Check sheet for the modelled part. Datum: model origin and axes. Units: mm. Face numbers are marked on the shaded views. A direction names the side the tool comes from. Give positions to 0.01 mm unless a question says otherwise; leave off trailing zeros. Order: outer loops, then holes, each group sorted by start corner. A loop starts at its lowest first (then second) coordinate and runs counter-clockwise, first axis right, second up. Notation, with made-up numbers: (-33, 85.5) - (-14, 85.5) arc R18 ccw to (-14, 116.5) - close; hole circle Ø11 at (-33.75, 56.5). An arc over 180 degrees is marked (long way). Answer in a Markdown table with one row per item.
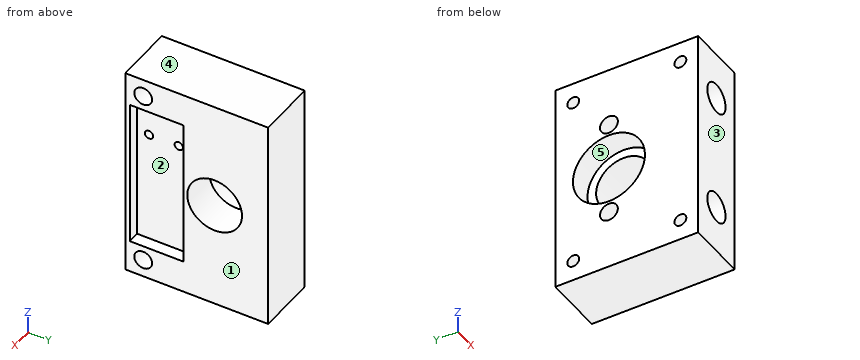
from build123d import *

# Parameters (mm, degrees)
SKETCH_1_W           = 36
SKETCH_1_H           = 24
EXTRUDE_1_DEPTH      = 10
SKETCH_2_R           = 6.05
CUT_EXTRUDE_1_DEPTH  = 4
SKETCH_3_R           = 4.6
CUT_EXTRUDE_2_DEPTH  = 7
SKETCH_5_R           = 2.5
CUT_EXTRUDE_4_DEPTH  = 8
SKETCH_7_W           = 25
SKETCH_7_H           = 9
CUT_EXTRUDE_5_DEPTH  = 2
SKETCH_8_R           = 1.5
CUT_EXTRUDE_6_DEPTH  = 5
SKETCH_9_R           = 1.5
CUT_EXTRUDE_7_DEPTH  = 5
SKETCH_11_R          = 1
CUT_EXTRUDE_9_DEPTH  = 3
SKETCH_13_R          = 0.7
CUT_EXTRUDE_10_DEPTH = 5


with BuildPart() as part:
    # 草图1 → 凸台-拉伸1 (new body)
    with BuildSketch(Plane(origin=(0, 0, 0), x_dir=(0, 0, -1), z_dir=(1, 0, 0))):
        with Locations((18, -12)):
            Rectangle(SKETCH_1_W, SKETCH_1_H)
    extrude(amount=EXTRUDE_1_DEPTH)

    # 草图2 → 切除-拉伸1 (cut)
    with BuildSketch(Plane.ZY):
        with Locations((-18, -9)):
            Circle(SKETCH_2_R)
    extrude(amount=-CUT_EXTRUDE_1_DEPTH, mode=Mode.SUBTRACT)

    # 草图3 → 切除-拉伸2 (cut, through all)
    with BuildSketch(Plane.ZY.offset(-4)):
        with Locations((-18, -9)):
            Circle(SKETCH_3_R)
    extrude(amount=-CUT_EXTRUDE_2_DEPTH, mode=Mode.SUBTRACT)

    # 草图5 → 切除-拉伸4 (cut)
    with BuildSketch(Plane(origin=(0, -24, 0), x_dir=(-1, 0, 0), z_dir=(0, -1, 0))):
        with Locations((-5, 28)):
            Circle(SKETCH_5_R)
        with Locations((-5, 8)):
            Circle(SKETCH_5_R)
    extrude(amount=-CUT_EXTRUDE_4_DEPTH, mode=Mode.SUBTRACT)

    # 草图7 → 切除-拉伸5 (cut)
    with BuildSketch(Plane(origin=(10, 0, 0), x_dir=(0, 0, -1), z_dir=(1, 0, 0))):
        with Locations((18, -18.75)):
            Rectangle(SKETCH_7_W, SKETCH_7_H)
    extrude(amount=-CUT_EXTRUDE_5_DEPTH, mode=Mode.SUBTRACT)

    # 草图8 → 切除-拉伸6 (cut)
    with BuildSketch(Plane.ZY):
        with Locations((-10, -9)):
            Circle(SKETCH_8_R)
        with Locations((-26, -9)):
            Circle(SKETCH_8_R)
    extrude(amount=-CUT_EXTRUDE_6_DEPTH, mode=Mode.SUBTRACT)

    # 草图9 → 切除-拉伸7 (cut)
    with BuildSketch(Plane(origin=(10, 0, 0), x_dir=(0, 0, -1), z_dir=(1, 0, 0))):
        with Locations((3, -21)):
            Circle(SKETCH_9_R)
        with Locations((33, -21)):
            Circle(SKETCH_9_R)
    extrude(amount=-CUT_EXTRUDE_7_DEPTH, mode=Mode.SUBTRACT)

    # 草图11 → 切除-拉伸9 (cut)
    with BuildSketch(Plane.ZY):
        with Locations((-32.5, -3)):
            Circle(SKETCH_11_R)
        with Locations((-32.5, -21)):
            Circle(SKETCH_11_R)
        with Locations((-3.5, -21)):
            Circle(SKETCH_11_R)
        with Locations((-3.5, -3)):
            Circle(SKETCH_11_R)
    extrude(amount=-CUT_EXTRUDE_9_DEPTH, mode=Mode.SUBTRACT)

    # 草图13 → 切除-拉伸10 (cut)
    with BuildSketch(Plane(origin=(8, 0, 0), x_dir=(0, 0, -1), z_dir=(1, 0, 0))):
        with Locations((11.5, -16.25)):
            Circle(SKETCH_13_R)
        with Locations((11.5, -21.25)):
            Circle(SKETCH_13_R)
    extrude(amount=-CUT_EXTRUDE_10_DEPTH, mode=Mode.SUBTRACT)


solid = part.part
(1) Gauge pin test, flat ends, axial feed: P1, Ø1.8, axis at y = -3, z = -32.5, coming from the -X side; P2, Ø1.8, axis at y = -21, z = -32.5, coming from the +X side; P3, Ø1.5, axis at x = 4, z = -29, coming from the -Y side. Record the tip position at first contact, or that the pin passes through.
Geometry says:
| item | result |
|---|---|
| P1 | x = 3 |
| P2 | x = 5 |
| P3 | y = -16 |
(2) Mould release check, pull along Y, two halves, no side actions. Record for the marked faces 3, 4 and 5: pulls with the +Y half, pulls with the -Y half, needs draft (parallel to the pull), parting line crosses it, or undercut.
Geometry says:
| item | result |
|---|---|
| face 3 | pulls with the -Y half |
| face 4 | needs draft |
| face 5 | undercut |
(3) Cross-section at A-A, the plane x = 8.5. Record the cut outline in (y, z).
Geometry says:
| item | result |
|---|---|
| outline | (-24, -36) - (0, -36) - (0, 0) - (-24, 0) - close; hole (-23.25, -30.5) - (-14.25, -30.5) - (-14.25, -5.5) - (-23.25, -5.5) - close; hole circle Ø3 at (-21, -33); hole circle Ø3 at (-21, -3); hole circle Ø9.2 at (-9, -18) |
(4) Cross-section at D-D, the plane z = -20. Record the cut outline in (x, y), then the cut area to 3 significant figures.
Geometry says:
| item | result |
|---|---|
| outline | (0, -24) - (10, -24) - (10, -23.25) - (8, -23.25) - (8, -14.25) - (10, -14.25) - (10, -13.14) - (4, -13.14) - (4, -14.71) - (0, -14.71) - close; (0, -3.29) - (4, -3.29) - (4, -4.86) - (10, -4.86) - (10, 0) - (0, 0) - close |
| area | 127 mm² |
(5) Cross-section at C-C, the plane y = -7. Record the cut outline in (x, z), then the cut area to 3 significant figures.
Geometry says:
| item | result |
|---|---|
| outline | (0, -36) - (10, -36) - (10, -22.14) - (4, -22.14) - (4, -23.71) - (0, -23.71) - close; (0, -12.29) - (4, -12.29) - (4, -13.86) - (10, -13.86) - (10, 0) - (0, 0) - close |
| area | 265 mm² |
(6) Thickness scan on L1, parallel to Y at x = 5.45, z = -11.5; L2, parallel to Y at x = 8.8, z = -3; L3, parallel to Y at x = 2, z = -18. Record the ranges inside material, lowest first.
Geometry says:
| item | result |
|---|---|
| L1 | -24 to -21.95, -20.55 to -16.95, -15.55 to 0 |
| L2 | -24 to -22.5, -19.5 to 0 |
| L3 | -24 to -15.05, -2.95 to 0 |
(7) Access from +Z, -Z, +X, -X, +Y, -Y to the whole of each face (thin tool, end or side, straight path). Record for the marked faces 1 and 2.
Geometry says:
| item | result |
|---|---|
| face 1 | +Z, -Z, +X, +Y, -Y |
| face 2 | +X |
(8) Cross-section at B-B, the plane x = 3.5. Record the cut outline in (y, z), then the cut area to 3 significant figures.
Geometry says:
| item | result |
|---|---|
| outline | (-24, -36) - (0, -36) - (0, 0) - (-24, 0) - (-24, -6) - (-16, -6) - (-16, -10) - (-24, -10) - (-24, -26) - (-16, -26) - (-16, -30) - (-24, -30) - close; hole circle Ø1.4 at (-21.25, -11.5); hole circle Ø1.4 at (-16.25, -11.5); hole circle Ø12.1 at (-9, -18); hole circle Ø3 at (-9, -26); hole circle Ø3 at (-9, -10) |
| area | 668 mm² |
